```python
from build123d import *
from build123d.topology import SkipClean

# Parameters (mm, degrees)
SKETCH1_R           = 1.25
SKETCH1_R_2         = 1.5
BOSS_EXTRUDE2_DEPTH = 4
SKETCH2_R           = 7.5
BOSS_EXTRUDE3_DEPTH = 2
SKETCH3_R           = 1.5
BOSS_EXTRUDE4_DEPTH = 2
SKETCH4_R           = 2.5
CUT_EXTRUDE1_DEPTH  = 4
SKETCH5_R           = 1
CUT_EXTRUDE2_DEPTH  = 30.412412346
SKETCH6_R           = 3.75
CUT_EXTRUDE3_DEPTH  = 1
CUT_EXTRUDE4_DEPTH  = 30.412412346
FILLET2_R           = 5
FILLET3_R           = 5
CHAMFER1_SIZE       = 0.2


with BuildPart() as part:
    # Sketch1 → Boss-Extrude2 (new body)
    with BuildSketch(Plane(origin=(0, 0, 0), x_dir=(1, 0, 0), z_dir=(0, 1, 0))):
        with BuildLine():
            ThreePointArc((24, -3.8), (27.8, 0), (24, 3.8))
            Line((24, 3.8), (6.466065264, 3.8))
            ThreePointArc((6.466065264, 3.8), (-7.5, 0), (6.466065264, -3.8))
            Line((6.466065264, -3.8), (24, -3.8))
        make_face()
        with Locations(Location((8.75, 0, 0), (0, 0, 270))):
            Circle(SKETCH1_R, mode=Mode.SUBTRACT)
        with Locations(Location((20, 0, 0), (0, 0, 270))):
            Circle(SKETCH1_R_2, mode=Mode.SUBTRACT)
        with Locations(Location((24, 0, 0), (0, 0, 270))):
            Circle(SKETCH1_R_2, mode=Mode.SUBTRACT)
    extrude(amount=BOSS_EXTRUDE2_DEPTH)

    # Sketch2 → Boss-Extrude3 (add)
    with BuildSketch(Plane(origin=(0, 4, 0), x_dir=(1, 0, 0), z_dir=(0, 1, 0))):
        with Locations(Location((0, 0, 0), (0, 0, 30.442052037))):
            Circle(SKETCH2_R)
    extrude(amount=BOSS_EXTRUDE3_DEPTH)

    # Sketch3 → Boss-Extrude4 (add)
    with BuildSketch(Plane(origin=(0, 4, 0), x_dir=(1, 0, 0), z_dir=(0, 1, 0))):
        with BuildLine():
            Line((24, 2.75), (20, 2.75))
            ThreePointArc((20, 2.75), (17.25, 0), (20, -2.75))
            Line((20, -2.75), (24, -2.75))
            ThreePointArc((24, -2.75), (26.75, 0), (24, 2.75))
        make_face()
        with Locations(Location((20, 0, 0), (0, 0, 270))):
            Circle(SKETCH3_R, mode=Mode.SUBTRACT)
        with Locations(Location((24, 0, 0), (0, 0, 270))):
            Circle(SKETCH3_R, mode=Mode.SUBTRACT)
    extrude(amount=BOSS_EXTRUDE4_DEPTH)

    # Sketch4 → Cut-Extrude1 (cut)
    with BuildSketch(Plane(origin=(0, 6, 0), x_dir=(1, 0, 0), z_dir=(0, 1, 0))):
        with Locations(Location((0, 0, 0), (0, 0, 270))):
            Circle(SKETCH4_R)
    extrude(amount=-CUT_EXTRUDE1_DEPTH, mode=Mode.SUBTRACT)

    # Sketch5 → Cut-Extrude2 (cut, through all)
    with BuildSketch(Plane(origin=(0, 0, 0), x_dir=(-1, 0, 0), z_dir=(0, -1, 0))):
        with Locations(Location((0, 0, 0), (0, 0, 90))):
            Circle(SKETCH5_R)
    extrude(amount=-CUT_EXTRUDE2_DEPTH, mode=Mode.SUBTRACT)

    # Sketch6 → Cut-Extrude3 (cut)
    with BuildSketch(Plane(origin=(0, 0, 0), x_dir=(-1, 0, 0), z_dir=(0, -1, 0))):
        with Locations(Location((0, 0, 0), (0, 0, 90))):
            Circle(SKETCH6_R)
    extrude(amount=-CUT_EXTRUDE3_DEPTH, mode=Mode.SUBTRACT)

    # Sketch7 → Cut-Extrude4 (cut, through all)
    with SkipClean():  # the faces are left unmerged after this step: merging them gives an invalid solid
        with BuildSketch(Plane(origin=(0, 0, 0), x_dir=(-1, 0, 0), z_dir=(0, -1, 0))):
            Polygon((-8.75, 0), (-8.75, -0.5), (10.38522601, -0.5), (10.38522601, 0.5), (-8.75, 0.5), align=None)
        extrude(amount=-CUT_EXTRUDE4_DEPTH, mode=Mode.SUBTRACT)
    add(part.part.scale(1), mode=Mode.REPLACE)  # the faces are merged on a copy

    # Fillet2
    fillet2_edges = [part.edges().sort_by_distance(p)[0] for p in [
        (6.466065264, 2, -3.8),
    ]]
    fillet(fillet2_edges, radius=FILLET2_R)

    # Fillet3
    # the kernel refuses this fillet: 5 mm, written as the material it adds along each edge
    with BuildSketch(Plane(origin=(6.466065264, 0, 3.8), x_dir=(-0.6100819962106524, 0, 0.792338285014441), z_dir=(0, 1, 0))) as fillet3_piece_1:
        with BuildLine():
            CenterArc((2.490518722, 4.961081765), FILLET3_R, 217.595432061, 45.251187916)
            Line((-1.471172703, 1.910671784), (0, 0))
            ThreePointArc((0, 0), (0.933944521, 0.058377352), (1.867889042, 0))
        make_face()
    extrude(amount=4)

    # Chamfer1
    chamfer1_edges = [part.edges().sort_by_distance(p)[0] for p in [
        (0, 6, -2.5),
        (0, 6, 2.5),
    ]]
    chamfer(chamfer1_edges, length=CHAMFER1_SIZE)


solid = part.part
```
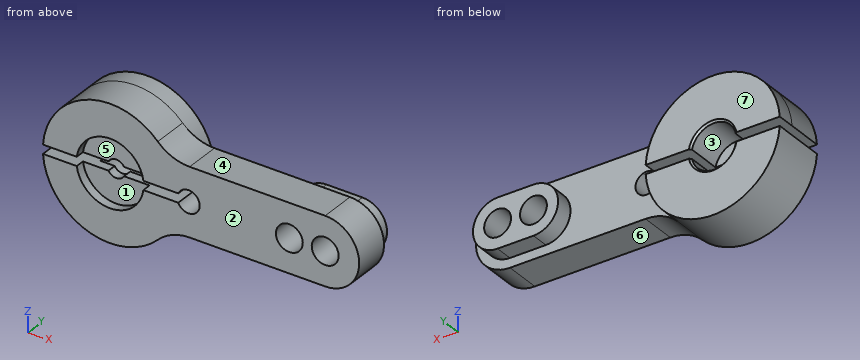
Work out the finished part from the listing and answer in its coordinate system (mm). Face numbers are marked on the shaded views. A direction names the side the tool comes from. Round coordinates to 2 decimals unless told otherwise and drop trailing zeros. Write each loop counter-clockwise with the first axis right and the second up, starting at its lowest first coordinate (ties: lowest second). Pieces come first, ordered by that corner, then holes.
1) A cutting plane is placed at D-D on y = 2.75. Determine the outline of the cut face in (x, z), and give its area (3 significant figures).
2) Which of the six approach directions +Z, -Z, +X, -X, +Y, -Y give full straight-line access (tool end or side, diameter ignored) to the marked faces 1, 2, 3 and 4?
3) Consider probe 1 along X at (y, z) = (2.5, 0); probe 2 along X at (y, z) = (4.5, 0); probe 3 along Z at (x, y) = (8.75, 2.75). Determine where each line is inside the solid, lowest interval first.
4) Determine the mould class of the marked faces 5, 6 and 7 for opening direction Z: pulls with the +Z half, pulls with the -Z half, needs draft (parallel to the pull), parting line crosses it, or undercut.
5) A cutting plane is placed at A-A on y = 4.6. Determine the outline of the cut face in (x, z), and give its area (3 significant figures).
6) A cutting plane is placed at C-C on z = 0. Determine the outline of the cut face in (x, y), and give its area (3 significant figures).
7) A cutting plane is placed at B-B on x = 0. Determine the outline of the cut face in (y, z), and give its area (3 significant figures).
8) Flat-ended cylindrical pins translate along their axes: P1, Ø1.2, axis at x = 15.5, y = 1.5, coming from the +Z side; P2, Ø1.8, axis at x = 2.5, y = 2.5, coming from the -Z side; P3, Ø3, axis at x = 13, y = 2, coming from the -Z side. Find the tip coordinate at first contact, or state that the pin passes through.
Entries:
1. outline: (-7.48, -0.5) arc R7.5 ccw to (5.33, -5.28) arc R5 cw to (8.88, -3.8) - (24, -3.8) arc R3.8 ccw to (24, 3.8) - (8.88, 3.8) arc R5 cw to (5.33, 5.28) arc R7.5 ccw to (-7.48, 0.5) - (-2.45, 0.5) arc R2.5 cw to (2.45, 0.5) - (7.6, 0.5) arc R1.25 cw (long way) to (7.6, -0.5) - (2.45, -0.5) arc R2.5 cw to (-2.45, -0.5) - close; hole circle Ø3 at (20, 0); hole circle Ø3 at (24, 0)
1. area: 280 mm2
2. face 1: -Y
2. face 2: +Z, -Z, +X, -X, -Y
2. face 3: +Y
2. face 4: +Z, +X, +Y, -Y
3. probe 1: x = 10 to 18.5, 21.5 to 22.5, 25.5 to 27.8
3. probe 2: x = 17.25 to 18.5, 21.5 to 22.5, 25.5 to 26.75
3. probe 3: z = -3.8 to -1.25, 1.25 to 3.8
4. face 5: undercut
4. face 6: pulls with the -Z half
4. face 7: needs draft
5. outline: (-7.48, -0.5) arc R7.5 ccw to (7.48, -0.5) - (2.45, -0.5) arc R2.5 cw to (-2.45, -0.5) - close; (-7.48, 0.5) - (-2.45, 0.5) arc R2.5 cw to (2.45, 0.5) - (7.48, 0.5) arc R7.5 ccw to start; (20, -2.75) - (24, -2.75) arc R2.75 ccw to (24, 2.75) - (20, 2.75) arc R2.75 ccw to start; hole circle Ø3 at (20, 0); hole circle Ø3 at (24, 0)
5. area: 179 mm2
6. outline: (10, 0) - (18.5, 0) - (18.5, 6) - (17.25, 6) - (17.25, 4) - (10, 4) - close; (21.5, 0) - (22.5, 0) - (22.5, 6) - (21.5, 6) - close; (25.5, 0) - (27.8, 0) - (27.8, 4) - (26.75, 4) - (26.75, 6) - (25.5, 6) - close
6. area: 54.2 mm2
7. outline: (0, -7.5) - (6, -7.5) - (6, -2.7) - (5.8, -2.5) - (2, -2.5) - (2, -1) - (1, -1) - (1, -3.75) - (0, -3.75) - close; (0, 3.75) - (1, 3.75) - (1, 1) - (2, 1) - (2, 2.5) - (5.8, 2.5) - (6, 2.7) - (6, 7.5) - (0, 7.5) - close
7. area: 60.5 mm2
8. P1: stops at z = 3.8
8. P2: stops at z = -7.33
8. P3: stops at z = -3.8
